Geometry check sheet. Reference: the model listing, model coordinates, mm. Face numbers are marked on the shaded views. A direction names the side the tool comes from. Give positions to 0.01 mm unless a question says otherwise; leave off trailing zeros. Order: outer loops, then holes, each group sorted by start corner. A loop starts at its lowest first (then second) coordinate and runs counter-clockwise, first axis right, second up.
Autodesk Inventor part; units mm, degrees
ref_plane "YZ Plane" through (0, 0, 0) normal (1, 0, 0) x (0, 1, 0)
ref_plane "XZ Plane" through (0, 0, 0) normal (0, 1, 0) x (-1, 0, 0)
ref_plane "XY Plane" through (0, 0, 0) normal (0, 0, 1) x (1, 0, 0)
sketch "Sketch1" plane through (0, 0, 0) normal (0, 1, 0) x (-1, 0, 0)
  line L0 (0, 0) -> (-152.4, 0)
  line L1 (-152.4, 0) -> (-152.4, -76.2)
  line L2 (-152.4, -76.2) -> (0, -76.2)
  line L3 (0, -76.2) -> (0, 0)
  dimension "d0" = 152.4
  dimension "d1" = 76.2
extrude "Extrusion1" add sketch "Sketch1" along normal blind 76.2
shell "Shell1" thickness 7.62 removed faces 1 at (101.6, 76.2, -25.4)
sketch "Sketch2" plane through (0, 0, -76.2) normal (-1, 0, 0) x (0, 0, 1)
  line L0 (0, 0) -> (0, 76.2)
  line L1 (0, 76.2) -> (68.58, 76.2)
  line L2 (68.58, 76.2) -> (68.58, 7.62)
  line L3 (68.58, 7.62) -> (0, 7.62)
  line L4 (0, 7.62) -> (0, 76.2)
  line L5 (0, 0) -> (76.2, 0)
  line L6 (76.2, 0) -> (76.2, 76.2)
  point P0 (7.62, 76.2)
  dimension "d5" = 7.62
  dimension "d6" = 7.62
  dimension "d7" = 7.62
extrude "Extrusion2" cut sketch "Sketch2" against normal up to surface (144.78 mm away)
sketch "Sketch3" plane through (0, 7.62, -7.62) normal (0, 1, 0) x (1, 0, 0)
  circle A0 centre (12.7, 11.43) radius 3.175
  line L0 (0, 0) -> (0, 68.58)
  line L1 (0, -7.62) -> (152.4, -7.62)
  dimension "d10" = 6.35
  dimension "d11" = 12.7
  dimension "d12" = 19.05
extrude "Extrusion3" cut sketch "Sketch3" against normal blind 25.4
properties part number "lift box"
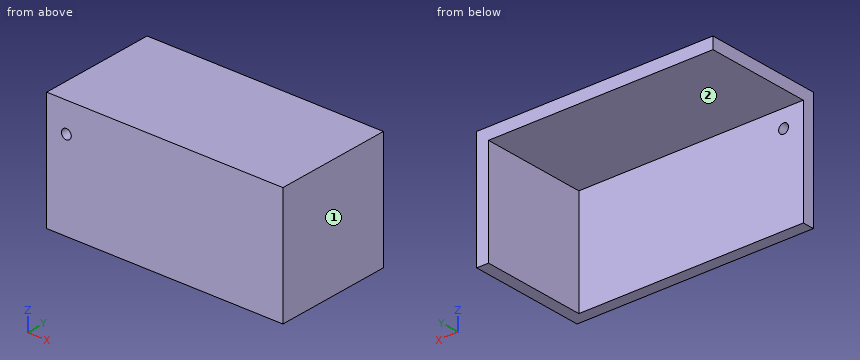
Item 1: Sectioned sample at C-C (x = 41). Enter the section's corners in (y, z), and give its area (3 significant figures).
Reported:
outline: (0, -76.2) - (7.62, -76.2) - (7.62, -7.62) - (76.2, -7.62) - (76.2, 0) - (0, 0) - close
area: 1,100 mm2
Item 2: Sectioned sample at A-A (x = 12.7). Enter the section's corners in (y, z) (3 decimals).
Reported:
outline: (0, -76.2) - (7.62, -76.2) - (7.62, -22.225) - (0, -22.225) - close; (0, -15.875) - (7.62, -15.875) - (7.62, -7.62) - (76.2, -7.62) - (76.2, 0) - (0, 0) - close
Item 3: Sectioned sample at B-B (z = -19.05). Enter the section's corners in (x, y) (3 decimals), and give its area (3 significant figures).
Reported:
outline: (0, 0) - (9.525, 0) - (9.525, 7.62) - (0, 7.62) - close; (15.875, 0) - (152.4, 0) - (152.4, 76.2) - (144.78, 76.2) - (144.78, 7.62) - (15.875, 7.62) - close
area: 1,640 mm2
Item 4: Scan lines: L1, parallel to X at y = 2.5, z = -19.05 (3 decimals); L2, parallel to Z at x = 113, y = 39.5; L3, parallel to X at y = 37.5, z = -13. Record each from-to range of solid material in increasing order.
Reported:
L1: x = 0 to 9.525, 15.875 to 152.4
L2: z = -7.62 to 0
L3: x = 144.78 to 152.4
Item 5: Set-up check for the marked faces 1 and 2: record each of +Z, -Z, +X, -X, +Y, -Y from which the full face is reachable in a straight line by a thin tool's end or side.
Reported:
face 1: +Z, -Z, +X, +Y, -Y
face 2: -Z, -X, +Y
Item 6: Sectioned sample at D-D (y = 65). Enter the section's corners in (x, z), and give its area (3 significant figures).
Reported:
outline: (0, -7.62) - (144.78, -7.62) - (144.78, -76.2) - (152.4, -76.2) - (152.4, 0) - (0, 0) - close
area: 1,680 mm2
Item 7: Gauge pin test, flat ends, axial feed: pin 1 (8 mm diameter, centred on y = 27.5, z = -13.5, fed in from -X); pin 2 (2 mm diameter, centred on x = 82.5, y = 49, fed in from +Z); pin 3 (1.5 mm diameter, centred on x = 36, z = -52.5, fed in from +Y); pin 4 (1 mm diameter, centred on x = 123, y = 56, fed in from -Z). Record the tip position at first contact, or that the pin passes through.
Reported:
pin 1: stops at x = 144.78
pin 2: stops at z = 0
pin 3: stops at y = 7.62
pin 4: stops at z = -7.62
